Here's how the part is built. I have some questions about the finished solid (model axes, mm). A direction names the side the tool comes from. Give positions to 0.01 mm unless a question says otherwise; leave off trailing zeros. Loops run counter-clockwise (first coordinate to the right, second up) from the corner with the lowest first, then second, coordinate; pieces in that order, holes last. Notation, with made-up numbers: (37.25, 54.5) - (54.25, 54.5) arc R19 ccw to (54.25, 83.5) - close; hole circle Ø1 at (32.5, 11). An arc over 180 degrees is marked (long way). Use one line per item in the form item = value.
from build123d import *

# Parameters (mm, degrees)
SKETCH_3_W      = 153.07917742657742
SKETCH_3_H      = 84.09905426521841
EXTRUDE_3_DEPTH = 10
SKETCH_4_R      = 5.999999999999998
SKETCH_4_R_2    = 6.000000000000017
SKETCH_4_R_3    = 6
EXTRUDE_4_DEPTH = 65
SKETCH_5_R      = 30.920810944079943
SKETCH_5_R_2    = 27.999999999999996
SKETCH_5_R_3    = 30.50629910833158
SKETCH_5_R_4    = 31.42305288564662
EXTRUDE_5_DEPTH = 10
FILLET_1_R      = 10
SKETCH_6_W      = 249.99999999999997
SKETCH_6_H      = 103.3253548332911
EXTRUDE_6_DEPTH = 3
SKETCH_7_W      = 111.7598891408415
SKETCH_7_H      = 103.3253548332911
EXTRUDE_7_DEPTH = 20
EXTRUDE_8_DEPTH = 30


with BuildPart() as part:
    # 草图3 → 凸台-拉伸3 (new body)
    with BuildSketch(Plane(origin=(0, 0, 0), x_dir=(1, 0, 0), z_dir=(0, 1, 0))):
        Polygon((0, 0), (249.99999999999997, 0), (249.99999999999997, -249.99999999999997), (3.062e-14, -249.99999999999997), align=None)
        with Locations((123.87065697506361, -146.07290630710244)):
            Rectangle(SKETCH_3_W, SKETCH_3_H, mode=Mode.SUBTRACT)
    extrude(amount=EXTRUDE_3_DEPTH)

    # 草图4 → 凸台-拉伸4 (add)
    with BuildSketch(Plane(origin=(0, 0, 0), x_dir=(1, 0, 0), z_dir=(0, 1, 0))):
        with Locations(Location((11.90907445269146, -61.60166288737722, 0), (0, 0, 270))):
            Circle(SKETCH_4_R)
        with Locations(Location((231.3648567656165, -61.60166288737722, 0), (0, 0, 270))):
            Circle(SKETCH_4_R_2)
        with Locations(Location((231.3648567656165, -186.93529856387, 0), (0, 0, 270))):
            Circle(SKETCH_4_R_2)
        with Locations(Location((11.90907445269146, -186.93529856387, 0), (0, 0, 270))):
            Circle(SKETCH_4_R_3)
    extrude(amount=-EXTRUDE_4_DEPTH)

    # 草图5 → 凸台-拉伸5 (add)
    # profile 1 of 3: a face of its own
    with BuildSketch(Plane(origin=(0, 10, 0), x_dir=(1, 0, 0), z_dir=(0, 1, 0))):
        with Locations(Location((32.374758545393455, -218.47190728143076, 0), (0, 0, 270))):
            Circle(SKETCH_5_R)
        with Locations(Location((32.374758545393455, -218.47190728143076, 0), (0, 0, 270))):
            Circle(SKETCH_5_R_2, mode=Mode.SUBTRACT)
    # profile 2 of 3: a face of its own
    with BuildSketch(Plane(origin=(0, 10, 0), x_dir=(1, 0, 0), z_dir=(0, 1, 0))):
        with Locations(Location((123.8146678424456, -218.47190728143076, 0), (0, 0, 84.187846026))):
            Circle(SKETCH_5_R_3)
        with Locations(Location((123.8146678424456, -218.47190728143076, 0), (0, 0, 270))):
            Circle(SKETCH_5_R_2, mode=Mode.SUBTRACT)
    # profile 3 of 3: a face of its own
    with BuildSketch(Plane(origin=(0, 10, 0), x_dir=(1, 0, 0), z_dir=(0, 1, 0))):
        with Locations(Location((213.22257915511878, -218.47190728143076, 0), (0, 0, 270))):
            Circle(SKETCH_5_R_4)
        with Locations(Location((213.22257915511878, -218.47190728143076, 0), (0, 0, 270))):
            Circle(SKETCH_5_R_2, mode=Mode.SUBTRACT)
    extrude(amount=EXTRUDE_5_DEPTH)

    # 圆角1
    # the kernel refuses this fillet: 10 mm, written as the material it takes off along each edge
    with BuildSketch(Plane(origin=(32.374758545393455, 20, 218.47190728143076), x_dir=(-2.5e-16, 0, 1), z_dir=(-1, 0, -2.5e-16))) as fillet_1_piece_1:
        with BuildLine():
            CenterArc((37.99999999999997, -7.062937229690062), FILLET_1_R, 135.06584304394207, 44.93415695605793)
            Line((27.99999999999997, -7.062937229690062), (27.799999999999983, -7.062937229690062))
            Line((27.799999999999983, -7.062937229690062), (27.80000000000001, 0))
            Line((27.80000000000001, 0), (28, 0.1999999999999993))
            ThreePointArc((28, 0.1999999999999993), (29.46040547203998, 0.1999999999999993), (30.77922716296152, 0.14125874459380228))
            Line((30.77922716296152, 0.14125874459380228), (30.920810944079932, 0))
        make_face()
    revolve(axis=Axis((32.374758545393455, 20, 218.47190728143076), (0, 1, 0)), mode=Mode.SUBTRACT)
    with BuildSketch(Plane(origin=(123.8146678424456, 20, 218.47190728143076), x_dir=(0, 0, 1), z_dir=(-1, 0, 0))) as fillet_1_piece_2:
        with BuildLine():
            CenterArc((37.99999999999997, -6.621513946689863), FILLET_1_R, 138.53584249731082, 41.464157502689176)
            Line((27.99999999999997, -6.621513946689863), (27.799999999999983, -6.621513946689863))
            Line((27.799999999999983, -6.621513946689863), (27.80000000000001, 0))
            Line((27.80000000000001, 0), (28, 0.1999999999999993))
            ThreePointArc((28, 0.1999999999999993), (29.253149554165788, 0.1999999999999993), (30.35642509049822, 0.13243027893379278))
            Line((30.35642509049822, 0.13243027893379278), (30.506299108331575, -3.55e-15))
        make_face()
    revolve(axis=Axis((123.8146678424456, 20, 218.47190728143076), (0, 1, 0)), mode=Mode.SUBTRACT)
    with BuildSketch(Plane(origin=(213.22257915511878, 20, 218.47190728143076), x_dir=(0, 0, 1), z_dir=(-1, 0, 0))) as fillet_1_piece_3:
        with BuildLine():
            CenterArc((37.99999999999997, -7.53284585365977), FILLET_1_R, 131.1242944649221, 48.87570553507791)
            Line((27.99999999999997, -7.53284585365977), (27.799999999999983, -7.53284585365977))
            Line((27.799999999999983, -7.53284585365977), (27.80000000000001, 0))
            Line((27.80000000000001, 0), (28, 0.1999999999999993))
            ThreePointArc((28, 0.1999999999999993), (29.711526442823327, 0.1999999999999993), (31.291513943359547, 0.15065691707319573))
            Line((31.291513943359547, 0.15065691707319573), (31.423052885646626, 0))
        make_face()
    revolve(axis=Axis((213.22257915511878, 20, 218.47190728143076), (0, 1, 0)), mode=Mode.SUBTRACT)

    # 草图6 → 凸台-拉伸6 (add)
    with BuildSketch(Plane(origin=(0, 10, 0), x_dir=(1, 0, 0), z_dir=(0, 1, 0))):
        with Locations((124.99999999999999, -51.66267741664555)):
            Rectangle(SKETCH_6_W, SKETCH_6_H)
    extrude(amount=EXTRUDE_6_DEPTH)

    # 草图7 → 凸台-拉伸7 (add)
    with BuildSketch(Plane(origin=(0, 0, 0), x_dir=(1, 0, 0), z_dir=(0, 1, 0))):
        with Locations((123.13733518098593, -51.66267741664555)):
            Rectangle(SKETCH_7_W, SKETCH_7_H)
    extrude(amount=EXTRUDE_7_DEPTH)

    # 草图8 → 凸台-拉伸8 (add)
    with BuildSketch(Plane(origin=(0, 20, 0), x_dir=(1, 0, 0), z_dir=(0, 1, 0))):
        with BuildLine():
            ThreePointArc((80.76980033741471, -53.36203223162917), (93.36972027799136, -80.59335577239693), (120.60104381875912, -93.19327571297359))
            ThreePointArc((120.60104381875912, -93.19327571297359), (124.13583776377907, -96.87481756004797), (127.670631708799, -93.19327571297359))
            ThreePointArc((127.670631708799, -93.19327571297359), (154.90195524956675, -80.59335577239695), (167.50187519014344, -53.3620322316292))
            ThreePointArc((167.50187519014344, -53.3620322316292), (171.18341703721785, -49.82723828660922), (167.50187519014344, -46.29244434158925))
            ThreePointArc((167.50187519014344, -46.29244434158925), (154.90195524956675, -19.06112080082149), (127.670631708799, -6.461200860244869))
            ThreePointArc((127.670631708799, -6.461200860244869), (124.13583776377907, -2.779659013170473), (120.60104381875912, -6.461200860244869))
            ThreePointArc((120.60104381875912, -6.461200860244869), (93.36972027799136, -19.061120800821513), (80.76980033741471, -46.29244434158928))
            ThreePointArc((80.76980033741471, -46.29244434158928), (77.08825849034031, -49.82723828660922), (80.76980033741471, -53.36203223162917))
        make_face()
    extrude(amount=EXTRUDE_8_DEPTH)


solid = part.part
(1) If we section it at D-D (y = -30): List the corners of the cut face in (x, z) for me.
Geometry says:
outline = circle Ø12 at (11.91, 61.6); circle Ø12 at (11.91, 186.94); circle Ø12 at (231.36, 61.6); circle Ø12 at (231.36, 186.94)
(2) If we section it at C-C (z = 23.5): List the corners of the cut face in (x, y) for me.
Geometry says:
outline = (0, 0) - (250, 0) - (250, 13) - (179.02, 13) - (179.02, 20) - (158.78, 20) - (158.78, 50) - (89.5, 50) - (89.5, 20) - (67.26, 20) - (67.26, 13) - (0, 13) - close
(3) For P1, Ø2, axis at x = 212, z = 130.5, coming from the +Y side; P2, Ø10, axis at x = 44, z = 164.5, coming from the -Y side; P3, Ø20, axis at x = 22.5, z = 43.5, coming from the +Y side, each with a flat end and sliding along its axis, tell me the tip position at first contact or that it passes through.
Geometry says:
P1 = 10
P2 = 0
P3 = 13
(4) If we section it at B-B (x = 159.5): List the corners of the cut face in (y, z) for me.
Geometry says:
outline = (0, 0) - (20, 0) - (20, 24.48) - (50, 24.48) - (50, 75.17) - (20, 75.17) - (20, 103.33) - (10, 103.33) - (10, 104.02) - (0, 104.02) - close; (0, 188.12) - (10, 188.12) - (10, 250) - (0, 250) - close
(5) Thinking about a two-plate mould opening in Z: for faces 1 (the cylindrical face through (77.09, 34.79, 49.75)), 2 (the flat face through (12, -65, 62)), 3 (the cylindrical face through (101.026, 14.93, 238.753)), 4 (the flat face through (123, 8, 0)), which applies, pulls with the +Z half, pulls with the -Z half, needs draft (parallel to the pull), parting line crosses it, or undercut?
Geometry says:
face_1 = parting line crosses it
face_2 = needs draft
face_3 = undercut
face_4 = pulls with the -Z half
(6) For faces 5 (the flat face through (123, 5, 104.023)), 6 (the cylindrical face through (93.07, 34.79, 80.29)), 7 (the flat face through (98, 20, 85)), 8 (the cylindrical face through (155.204, 34.79, 19.366)), 9 (the flat face through (179.017, 16, 52)), which set-ups out of +Z, -Z, +X, -X, +Y, -Y let a thin tool reach every point of the face, with its end or its side?
Geometry says:
face_5 = +Y, -Y
face_6 = +Z, -X, +Y
face_7 = +Y
face_8 = -Z, +X, +Y
face_9 = +Z, -Z, +X, +Y
(7) If I drill on probe 1 along Y at (x, z) = (183.5, 100); probe 2 along Z at (x, y) = (162, 12); probe 3 along X at (y, z) = (13.5, 21.5), over which ranges is the centre line in solid material (lowest first)?
Geometry says:
probe_1 = 0 to 13
probe_2 = 0 to 103.33
probe_3 = 67.26 to 179.02
(8) If we section it at A-A (z = 172.5): List the corners of the cut face in (x, y) for me.
Geometry says:
outline = (0, 0) - (47.33, 0) - (47.33, 10) - (0, 10) - close; (200.41, 0) - (250, 0) - (250, 10) - (200.41, 10) - close
